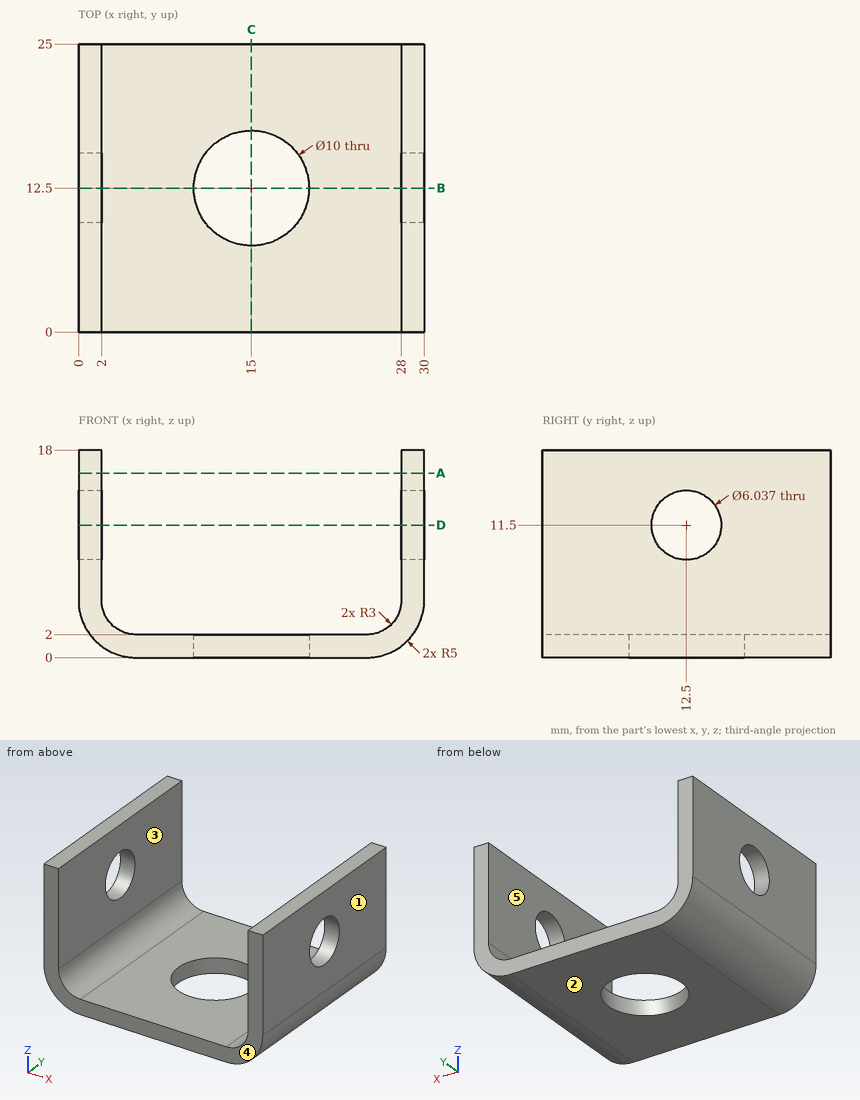
Can you work these out from the drawing? Everything is in mm from the part's minimum corner. A direction names the side the tool comes from. Coordinates: 2 decimals unless noted, no trailing zeros. Loops run counter-clockwise (first coordinate to the right, second up) from the corner with the lowest first, then second, coordinate; pieces in that order, holes last. Notation, with made-up numbers: (85, 40.25) - (108, 40.25) arc R20 cw to (108, 59.25) - close; hole circle Ø2 at (11.25, -36). An arc over 180 degrees is marked (long way). Use a Markdown table: item, result.
Item 1: I want a section at B-B on y = 12.5. Please give me the cut outline in (x, z).
Numbers:
| item | result |
|---|---|
| outline | (0, 5) arc R5 ccw to (5, 0) - (10, 0) - (10, 2) - (5, 2) arc R3 cw to (2, 5) - (2, 8.48) - (0, 8.48) - close; (0, 14.52) - (2, 14.52) - (2, 18) - (0, 18) - close; (20, 0) - (25, 0) arc R5 ccw to (30, 5) - (30, 8.48) - (28, 8.48) - (28, 5) arc R3 cw to (25, 2) - (20, 2) - close; (28, 14.52) - (30, 14.52) - (30, 18) - (28, 18) - close |
Item 2: If I drill on probe 1 along Y at (x, z) = (28.6, 11.5); probe 2 along X at (y, z) = (13, 7.75); probe 3 along Z at (x, y) = (9, 17.5), over which ranges is the centre line in solid material (lowest first)? Write a range as from..to.
Numbers:
| item | result |
|---|---|
| probe 1 | y = 0..9.48, 15.52..25 |
| probe 2 | x = 0..2, 28..30 |
| probe 3 | z = 0..2 |
Item 3: Will these pins go through, and if not, where does the flat tip stop? pin 1 (4 mm diameter, centred on x = 24, y = 17.5, fed in from +Z); pin 2 (8 mm diameter, centred on x = 13.5, y = 11.5, fed in from +Z); pin 3 (1.5 mm diameter, centred on x = 3.5, y = 16, fed in from +Z) (1 decimal); pin 4 (6 mm diameter, centred on x = 15, y = 12.5, fed in from +Z).
Numbers:
| item | result |
|---|---|
| pin 1 | stops at z = 2.17 |
| pin 2 | stops at z = 2 |
| pin 3 | stops at z = 3 |
| pin 4 | passes through |
Item 4: I want a section at A-A on z = 16. Please give me the cut outline in (x, y), and give its area (3 significant figures).
Numbers:
| item | result |
|---|---|
| outline | (0, 0) - (2, 0) - (2, 25) - (0, 25) - close; (28, 0) - (30, 0) - (30, 25) - (28, 25) - close |
| area | 100 mm2 |
Item 5: I want a section at C-C on x = 15. Please give me the cut outline in (y, z).
Numbers:
| item | result |
|---|---|
| outline | (0, 0) - (7.5, 0) - (7.5, 2) - (0, 2) - close; (17.5, 0) - (25, 0) - (25, 2) - (17.5, 2) - close |
Item 6: I want a section at D-D on z = 11.5. Please give me the cut outline in (x, y).
Numbers:
| item | result |
|---|---|
| outline | (0, 0) - (2, 0) - (2, 9.48) - (0, 9.48) - close; (0, 15.52) - (2, 15.52) - (2, 25) - (0, 25) - close; (28, 0) - (30, 0) - (30, 9.48) - (28, 9.48) - close; (28, 15.52) - (30, 15.52) - (30, 25) - (28, 25) - close |
Item 7: We'd pull the mould along X, two halves only. Please class the marked faces 1, 2 and 3: released by +X, released by -X, zero draft, split by the parting line, or undercut.
Numbers:
| item | result |
|---|---|
| face 1 | released by +X |
| face 2 | zero draft |
| face 3 | undercut |
Item 8: For the marked faces 4 and 5, which set-ups out of +Z, -Z, +X, -X, +Y, -Y let a thin tool reach every point of the face, with its end or its side?
Numbers:
| item | result |
|---|---|
| face 4 | +Z, -Z, +X, -X, -Y |
| face 5 | +Z, +Y, -Y |
